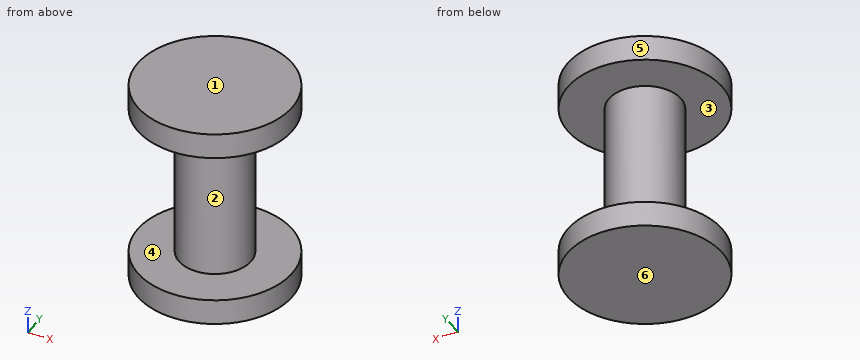
```python
from build123d import *

# Parameters (mm, degrees)
SKETCH_1_R           = 30
SKETCH_1_R_2         = 14
EXTRUDE_1_DEPTH      = 10
SKETCH_2_R           = 14
EXTRUDE_2_DEPTH      = 70
EXTRUDE_2_DEPTH_BACK = 10
SKETCH_3_R           = 30
SKETCH_3_R_2         = 14
EXTRUDE_3_DEPTH      = 10


with BuildPart() as part:
    # 草图1 → 凸台-拉伸1 (new body)
    with BuildSketch(Plane.XY):
        Circle(SKETCH_1_R)
        Circle(SKETCH_1_R_2, mode=Mode.SUBTRACT)
    extrude(amount=EXTRUDE_1_DEPTH)

    # 草图2 → 凸台-拉伸2 (add, two sides)
    with BuildSketch(Plane.XY.offset(10)) as extrude_2_sk:
        Circle(SKETCH_2_R)
    extrude(amount=EXTRUDE_2_DEPTH)
    extrude(extrude_2_sk.sketch, amount=-EXTRUDE_2_DEPTH_BACK)

    # 草图3 → 凸台-拉伸3 (add)
    with BuildSketch(Plane.XY.offset(80)):
        Circle(SKETCH_3_R)
        Circle(SKETCH_3_R_2, mode=Mode.SUBTRACT)
    extrude(amount=-EXTRUDE_3_DEPTH)


solid = part.part
```
Design review of the part built by this model. Coordinates are the model's own, in mm. Face numbers are marked on the shaded views. A direction names the side the tool comes from. Round coordinates to 2 decimals unless told otherwise and drop trailing zeros. Write each loop counter-clockwise with the first axis right and the second up, starting at its lowest first coordinate (ties: lowest second). Pieces come first, ordered by that corner, then holes. Notation, with made-up numbers: (15.25, 16) -> (20.25, 16) arc R17 cw to (20.25, 28) -> close; hole circle Ø2 at (76.5, 51). An arc over 180 degrees is marked (long way). Write item = value, one per line. Start each with the question number.
1) Take a section at D-D, the plane z = 32. State the section outline as (x, y) points, plus the area to 3 significant figures.
2) Wall thickness on probe 1 along Z at (x, y) = (-2, -19); probe 2 along X at (y, z) = (4, 21); probe 3 along X at (y, z) = (12.5, 30): over which ranges is each line inside the solid? List them lowest first. Write a range as from..to.
3) Tool access review of the marked faces 1 and 2: name each direction out of +Z, -Z, +X, -X, +Y, -Y from which nothing blocks a thin tool from reaching the whole face with its end or side.
4) Take a section at A-A, the plane y = 25. State the section outline as (x, z) points.
5) Take a section at B-B, the plane x = 0. State the section outline as (y, z) points.
6) Mouldability with a two-part tool opening along Z and no side actions: class the marked faces 3, 4, 5 and 6 as +Z half, -Z half, draft (parallel to the pull), parting line (faces both ways), or undercut.
7) Clearance check with flat-ended pins moving along their axes: pin 1 (5 mm diameter, centred on x = -3.5, z = 41, fed in from +Y); pin 2 (5 mm diameter, centred on x = 22, z = 70, fed in from -Y); pin 3 (12 mm diameter, centred on y = 2.5, z = 42, fed in from +X). State where each tip first meets the part, or that it passes through.
Results list:
q1.outline = circle Ø28 at (0, 0)
q1.area = 616 mm²
q2.probe_1 = 0..10, 70..80
q2.probe_2 = -13.42..13.42
q2.probe_3 = -6.3..6.3
q3.face_1 = +Z, +X, -X, +Y, -Y
q3.face_2 = none
q4.outline = (-16.58, 0) -> (16.58, 0) -> (16.58, 10) -> (-16.58, 10) -> close; (-16.58, 70) -> (16.58, 70) -> (16.58, 80) -> (-16.58, 80) -> close
q5.outline = (-30, 0) -> (30, 0) -> (30, 10) -> (14, 10) -> (14, 70) -> (30, 70) -> (30, 80) -> (-30, 80) -> (-30, 70) -> (-14, 70) -> (-14, 10) -> (-30, 10) -> close
q6.face_3 = undercut
q6.face_4 = undercut
q6.face_5 = draft
q6.face_6 = -Z half
q7.pin_1 = 13.96
q7.pin_2 = -22.8
q7.pin_3 = 14
